Autodesk Inventor part; units mm, degrees
ref_plane "YZ Plane" through (0, 0, 0) normal (1, 0, 0) x (0, 1, 0)
ref_plane "XZ Plane" through (0, 0, 0) normal (0, 1, 0) x (-1, 0, 0)
ref_plane "XY Plane" through (0, 0, 0) normal (0, 0, 1) x (1, 0, 0)
sketch "Sketch1" plane through (0, 0, 0) normal (0, 1, 0) x (-1, 0, 0)
  circle A0 centre (0, 0) radius 4
  dimension "d0" = 8
extrude "Extrusion1" add sketch "Sketch1" along normal blind 5
sketch "Sketch2" plane through (0, 5, 0) normal (0, 1, 0) x (1, 0, 0)
  circle A0 centre (0, 0) radius 2.5
  dimension "d3" = 5
extrude "Extrusion2" add sketch "Sketch2" along normal blind 35
sketch "Sketch3" plane through (0, 0, 0) normal (0, -1, 0) x (1, 0, 0)
  line L0 (2.8865, -0.0416) -> (1.4072, -2.5205)
  line L1 (1.4072, -2.5205) -> (-1.4792, -2.479)
  line L2 (-1.4792, -2.479) -> (-2.8865, 0.0416)
  line L3 (-2.8865, 0.0416) -> (-1.4072, 2.5205)
  line L4 (-1.4072, 2.5205) -> (1.4792, 2.479)
  line L5 (1.4792, 2.479) -> (2.8865, -0.0416)
  point P0 (0, 0)
  point P1 (0, 0)
  dimension "d6" = 2.5
extrude "Extrusion3" cut sketch "Sketch3" against normal blind 3
fillet "Fillet1" radius 0.5 1 edges at (4, 0, 0)
fillet "Fillet2" radius 0.5 2 edges at (-2.5, 5, 0) (-2.5, 40, 0)
properties part number "bulong5mm"
Design review of the part built by this model. Coordinates are the model's own, in mm. A direction names the side the tool comes from. Give positions to 0.01 mm unless a question says otherwise; leave off trailing zeros. Order: outer loops, then holes, each group sorted by start corner. A loop starts at its lowest first (then second) coordinate and runs counter-clockwise, first axis right, second up.
1. To check wall thickness, follow L1, parallel to Z at x = -1.5, y = 30; L2, parallel to Y at x = 0.75, z = -0.5; L3, parallel to Y at x = -3, z = 0.75. State the ranges of each line that lie inside material, in increasing order.
Solution:
L1: z = -2 to 2
L2: y = 3 to 40
L3: y = 0 to 5
2. Tool access review of faces 5 (the cylindrical face through (-0.54, 22.26, -2.44)), 6 (the flat face through (-2.17, 1.48, -1.24)), 7 (the flat face through (0, 40, 0)): name each direction out of +Z, -Z, +X, -X, +Y, -Y from which nothing blocks a thin tool from reaching the whole face with its end or side.
Solution:
face 5: +Y
face 6: -Y
face 7: +Z, -Z, +X, -X, +Y
3. For pin 1 Ø4 at (x, z) = (-1.5, -1.5) entering from -Y; pin 2 Ø2 at (y, z) = (11, -1.5) entering from -X; pin 3 Ø3 at (x, y) = (2.5, 9.5) entering from -Z, all flat-tipped, find the tip position at first contact; note any pin that passes through.
Solution:
pin 1: stops at y = 0
pin 2: stops at x = -2.45
pin 3: stops at z = -2.29
4. Add section A-A, the plane x = 0. State the section outline as (y, z) points.
Solution:
outline: (0, -3.5) arc R0.5 ccw to (0.5, -4) - (5, -4) - (5, -3) arc R0.5 cw to (5.5, -2.5) - (39.5, -2.5) arc R0.5 ccw to (40, -2) - (40, 2) arc R0.5 ccw to (39.5, 2.5) - (5.5, 2.5) arc R0.5 cw to (5, 3) - (5, 4) - (0.5, 4) arc R0.5 ccw to (0, 3.5) - (0, 2.5) - (3, 2.5) - (3, -2.5) - (0, -2.5) - close
5. Mouldability with a two-part tool opening along X and no side actions: class faces 1 (the flat face through (-2.16, 1.48, 1.26)), 2 (the cylindrical face through (0.867, 2.718, 3.905)), 3 (the flat face through (2, 0, -2)), 4 (the flat face through (2.17, 1.48, 1.24)) as +X half, -X half, draft (parallel to the pull), parting line (faces both ways), or undercut.
Solution:
face 1: undercut
face 2: parting line
face 3: draft
face 4: undercut
6. Add section B-B, the plane y = 36. State the section outline as (x, z) points, then the cut area to 3 significant figures.
Solution:
outline: circle Ø5 at (0, 0)
area: 19.6 mm2
